The listing builds one solid part. Answer for the finished solid, in the listing's coordinates (mm). A direction names the side the tool comes from. Round coordinates to 2 decimals unless told otherwise and drop trailing zeros. Write each loop counter-clockwise with the first axis right and the second up, starting at its lowest first coordinate (ties: lowest second). Pieces come first, ordered by that corner, then holes. Notation, with made-up numbers: (-36.5, -39.75) - (-11.5, -39.75) arc R11 ccw to (-11.5, -27.75) - close; hole circle Ø7 at (72.25, 80). An arc over 180 degrees is marked (long way). Use a Markdown table: item, result. Add a question column.
1) A tool of negligible diameter and unlimited length cuts with its end or side. For faces 5 (the flat face through (12, 0, 2)), 6 (the flat face through (23, 16.8, 14)), 7 (the flat face through (62.5, 13, 8)), 8 (the flat face through (54, 12.7, 14)), 9 (the flat face through (49, 18, 12)), from which of +Z, -Z, +X, -X, +Y, -Y can it reach the whole face along a straight path? Write none if from no direction.
2) A cutting plane is placed at D-D (y = 14.25). Give the vertices of the cut face in (x, z), then the cut area to 3 significant figures.
3) Determine the mould class of faces 1 (the cylindrical face through (10.654, 4.8, 1.622)), 2 (the cylindrical face through (42.6, 10, 1.6)), 3 (the flat face through (0, 17, 7)), 4 (the flat face through (24, 12, 0)) for opening direction X: +X half, -X half, draft (parallel to the pull), parting line (faces both ways), or undercut.
4) A cutting plane is placed at A-A (x = 9.7). Give the vertices of the cut face in (y, z).
5) A cutting plane is placed at B-B (y = 6.75). Give the vertices of the cut face in (x, z).
6) A cutting plane is placed at C-C (z = 5.25). Give the vertices of the cut face in (x, y), then the cut area to 3 significant figures.
7) Find the intervals of material crossed by probe 1 along Y at (x, z) = (9.7, 0.8); probe 2 along Z at (x, y) = (54, 9.25); probe 3 along Y at (x, z) = (38.5, 20), in increasing order. Write a range as from..to.
8) Each of these flat-tipped pins is pushed along its axis until it touches: P1, Ø3.5, axis at y = 14.5, z = 12.5, coming from the -X side; P2, Ø8.5, axis at x = 29, y = 12, coming from the +Z side; P3, Ø1, axis at y = 12, z = 19, coming from the -X side; P4, Ø1.8, axis at y = 18, z = 11, coming from the +X side. Where does it stop, or does it pass through?
```python
from build123d import *

# Parameters (mm, degrees)
F1_DEPTH = 3.2
F2_R     = 20
F3_DEPTH = 25
F4_R     = 1
F5_DEPTH = 25
F6_R     = 2.25
F7_DEPTH = 25
F9_DEPTH = 21


with BuildPart() as f1:
    # F0 (on Top) → F1 (new body)
    with BuildSketch(Plane.XY):
        Polygon((0, 0), (62.5, 0), (62.5, 16.3), (49, 16.3), (49, 20), (0, 20), align=None)
    extrude(amount=F1_DEPTH)

    # F2 (on face) → F3 (cut)
    with BuildSketch(Plane.XY.offset(3.2)):
        with Locations((42.349905, -10)):
            Circle(F2_R)
    extrude(amount=-F3_DEPTH, mode=Mode.SUBTRACT)

    # F4 (on face) → F5 (cut)
    with BuildSketch(Plane.XY.offset(3.2)):
        with Locations((9.7, 4.5)):
            Circle(F4_R)
    extrude(amount=-F5_DEPTH, mode=Mode.SUBTRACT)

    # F6 (on face) → F7 (cut)
    with BuildSketch(Plane.XY.offset(3.2)):
        with Locations((26.5, 6.75)):
            Circle(F6_R)
        with Locations((58.2, 6.75)):
            Circle(F6_R)
    extrude(amount=-F7_DEPTH, mode=Mode.SUBTRACT)

    # F8 (on face) → F9 (join)
    with BuildSketch(Plane.XY.offset(3.2)):
        Polygon((49, 20), (0, 20), (0, 16.8), (45.8, 16.8), (45.8, 12.7), (62.5, 12.7), (62.5, 16.3), (49, 16.3), align=None)
    extrude(amount=F9_DEPTH)


solid = f1.part
```
Entries:
| question | item | result |
|---|---|---|
| 1 | face 5 | +Z, -Z, +X, -X, -Y |
| 1 | face 6 | +Z, -X, -Y |
| 1 | face 7 | +Z, -Z, +X, +Y, -Y |
| 1 | face 8 | +Z, +X, -X, -Y |
| 1 | face 9 | +Z, -Z, +X, +Y |
| 2 | outline | (0, 0) - (62.5, 0) - (62.5, 24.2) - (45.8, 24.2) - (45.8, 3.2) - (0, 3.2) - close |
| 2 | area | 551 mm² |
| 3 | face 1 | undercut |
| 3 | face 2 | undercut |
| 3 | face 3 | -X half |
| 3 | face 4 | draft |
| 4 | outline | (0, 0) - (3.5, 0) - (3.5, 3.2) - (0, 3.2) - close; (5.5, 0) - (20, 0) - (20, 24.2) - (16.8, 24.2) - (16.8, 3.2) - (5.5, 3.2) - close |
| 5 | outline | (0, 0) - (24.25, 0) - (24.25, 3.2) - (0, 3.2) - close; (28.75, 0) - (31.42, 0) - (31.42, 3.2) - (28.75, 3.2) - close; (53.28, 0) - (55.95, 0) - (55.95, 3.2) - (53.28, 3.2) - close; (60.45, 0) - (62.5, 0) - (62.5, 3.2) - (60.45, 3.2) - close |
| 6 | outline | (0, 16.8) - (45.8, 16.8) - (45.8, 12.7) - (62.5, 12.7) - (62.5, 16.3) - (49, 16.3) - (49, 20) - (0, 20) - close |
| 6 | area | 219 mm² |
| 7 | probe 1 | y = 0..3.5, 5.5..20 |
| 7 | probe 2 | z = 0..3.2 |
| 7 | probe 3 | y = 16.8..20 |
| 8 | P1 | stops at x = 45.8 |
| 8 | P2 | stops at z = 3.2 |
| 8 | P3 | passes through |
| 8 | P4 | stops at x = 49 |
